from build123d import *

# Parameters (mm, degrees)
SKETCH2_R               = 15
SKETCH2_R_2             = 13
BOSS_EXTRUDE1_DEPTH     = 70
CUT_EXTRUDE1_DEPTH      = 74.143694192
CUT_EXTRUDE1_DEPTH_BACK = 74.143694192
SKETCH4_W               = 40
SKETCH4_H               = 35
BOSS_EXTRUDE2_DEPTH     = 4
SKETCH5_W               = 4
SKETCH5_H               = 35
BOSS_EXTRUDE4_DEPTH     = 40
SKETCH6_R               = 5
CUT_EXTRUDE2_DEPTH      = 101.39586407
FILLET3_R               = 17.5


with BuildPart() as part:
    # Sketch2 → Boss-Extrude1 (new body)
    with BuildSketch(Plane(origin=(0, 0, 0), x_dir=(1, 0, 0), z_dir=(0, 1, 0))):
        with Locations(Location((0, 0, 0), (0, 0, 270))):
            Circle(SKETCH2_R)
        with Locations(Location((0, 0, 0), (0, 0, 270))):
            Circle(SKETCH2_R_2, mode=Mode.SUBTRACT)
    extrude(amount=BOSS_EXTRUDE1_DEPTH)

    # Sketch3 → Cut-Extrude1 (cut, two sides: drawn at the far end of the back side and taken through both)
    with BuildSketch(Plane.XY.offset(-CUT_EXTRUDE1_DEPTH_BACK)):
        Polygon((-15, 52.679491924), (-15, 70), (15, 70), align=None)
    extrude(amount=CUT_EXTRUDE1_DEPTH + CUT_EXTRUDE1_DEPTH_BACK, mode=Mode.SUBTRACT)

    # Sketch4 → Boss-Extrude2 (add)
    with BuildSketch(Plane(origin=(-26.560889132, 46.004809472, 0), x_dir=(0.866025403784438, 0.5000000000000012, 0), z_dir=(-0.5000000000000012, 0.866025403784438, 0))):
        with Locations((30.669872981, 0)):
            Rectangle(SKETCH4_W, SKETCH4_H)
    extrude(amount=BOSS_EXTRUDE2_DEPTH)

    # Sketch5 → Boss-Extrude4 (add)
    with BuildSketch(Plane(origin=(-28.560889132, 49.468911087, 0), x_dir=(0.866025403784438, 0.5000000000000012, 0), z_dir=(-0.5000000000000011, 0.8660254037844379, 0))):
        with Locations((30.669872981, 0)):
            Rectangle(SKETCH5_W, SKETCH5_H)
    extrude(amount=BOSS_EXTRUDE4_DEPTH)

    # Sketch6 → Cut-Extrude2 (cut, through all)
    with BuildSketch(Plane(origin=(24.828838325, 14.334936491, 0), x_dir=(0, 0, 1), z_dir=(-0.8660254037844382, -0.5000000000000011, 0))):
        with Locations(Location((0, 82.121778265, 0), (0, 0, 270))):
            Circle(SKETCH6_R)
    extrude(amount=-CUT_EXTRUDE2_DEPTH, mode=Mode.SUBTRACT)

    # Fillet3
    fillet3_edges = [part.edges().sort_by_distance(p)[0] for p in [
        (-22, 99.444863729, 17.5),
        (-22, 99.444863729, -17.5),
    ]]
    fillet(fillet3_edges, radius=FILLET3_R - 0.0001)  # a hair under: the kernel refuses the full size


solid = part.part
Could you check a few things on this model? Use its own coordinates, in mm. A direction names the side the tool comes from. Round coordinates to 2 decimals unless told otherwise and drop trailing zeros. Order: outer loops, then holes, each group sorted by start corner. A loop starts at its lowest first (then second) coordinate and runs counter-clockwise, first axis right, second up.
Q1. Thinking about a two-plate mould opening in Y: for faces 4 (the face through (12.89, 34.03, -1.69)), 5 (the face through (-19.345, 94.901, -12.51)), 6 (the face through (-13.59, 80.88, 0.25)), which applies, released by +Y, released by -Y, zero draft, split by the parting line, or undercut?
Geometry says:
face 4: zero draft
face 5: released by +Y
face 6: undercut
Q2. I'm going to push flat-ended pins straight in: P1, Ø8, axis at y = 82, z = 0, coming from the -X side; P2, Ø1, axis at y = 88, z = -7.5, coming from the +X side; P3, Ø3, axis at x = 1, y = 12.5, coming from the -Z side. Where does each tip first touch, or does it pass through?
Geometry says:
P1: stops at x = -14.68
P2: stops at x = -12.79
P3: stops at z = -15
Q3. Imagine slicing it at D-D, the plane x = 5.5. List the corners of the cut face in (y, z) for me.
Geometry says:
outline: (0, -13.96) - (64.52, -13.96) - (64.52, -17.5) - (69.13, -17.5) - (69.13, 17.5) - (64.52, 17.5) - (64.52, 13.96) - (0, 13.96) - (0, 11.78) - (64.52, 11.78) - (64.52, -11.78) - (0, -11.78) - close
Q4. Please list where these lines run through material, in increasing order: probe 1 along X at (y, z) = (37, 0); probe 2 along Y at (x, z) = (-10, 7).
Geometry says:
probe 1: x = -15 to -13, 13 to 15
probe 2: y = 55.57 to 60.19, 74.66 to 82.66
Q5. Imagine slicing it at A-A, the plane x = -8.5. List the corners of the cut face in (y, z) for me, then the cut area to 3 significant figures.
Geometry says:
outline: (0, -12.36) - (56.43, -12.36) - (56.43, -17.5) - (61.05, -17.5) - (61.05, 17.5) - (56.43, 17.5) - (56.43, 12.36) - (0, 12.36) - (0, 9.84) - (56.43, 9.84) - (56.43, -9.84) - (0, -9.84) - close; (72.06, -17.5) - (80.06, -17.5) - (80.06, 17.5) - (72.06, 17.5) - close
area: 726 mm2
Q6. Imagine slicing it at C-C, the plane y = 60. List the corners of the cut face in (x, z) for me.
Geometry says:
outline: (-10.32, -17.5) - (-2.32, -17.5) - (-2.32, -14.82) arc R15 ccw (long way) to (-2.32, 14.82) - (-2.32, 17.5) - (-10.32, 17.5) - close; hole (-2.32, -12.79) arc R13 ccw (long way) to (-2.32, 12.79) - close
Q7. Which directions (+Z, -Z, +X, -X, +Y, -Y) give clear straight access to the entire face, cutting with the end or side of a thin tool? Please do faces 1 (the face through (-0.24, 61.2, 15.31)), 2 (the face through (7, 70, 0)), 3 (the face through (-11.64, 59.24, -0.25)).
Geometry says:
face 1: -Y
face 2: +Z, -Z, +Y
face 3: +Z, -Z, -X
Q8. Imagine slicing it at B-B, the plane z = -7. List the corners of the cut face in (x, y) for me.
Geometry says:
outline: (-23, 97.18) - (-3.73, 63.8) - (-19.32, 54.8) - (-17.32, 51.34) - (-13.27, 53.68) - (-13.27, 0) - (-10.95, 0) - (-10.95, 55.02) - (10.95, 67.66) - (10.95, 0) - (13.27, 0) - (13.27, 69) - (17.32, 71.34) - (15.32, 74.8) - (-0.27, 65.8) - (-19.54, 99.18) - close
